Check sheet for the drawn part. Datum: minimum x, y, z corner. Units: mm. A direction names the side the tool comes from. Round coordinates to 2 decimals unless told otherwise and drop trailing zeros. Write each loop counter-clockwise with the first axis right and the second up, starting at its lowest first coordinate (ties: lowest second). Pieces come first, ordered by that corner, then holes. Notation, with made-up numbers: M 71.5,81 L 81.5,81 A23 cw 81.5,108 Z; hole C -22.5,58 d11. An arc over 180 degrees is marked long. Answer in a Markdown table with one row per item. Add a question column.
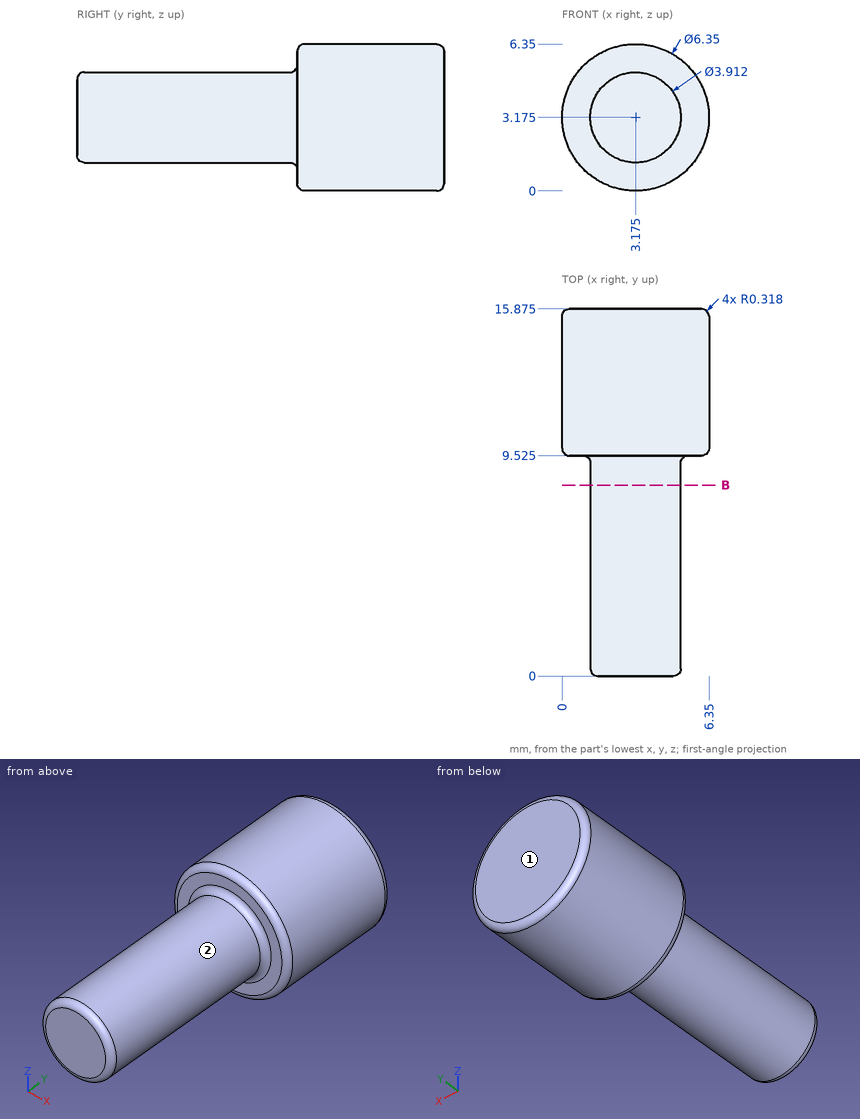
Item 1: Section check B-B, the plane y = 8.25. Record the boundary of the cut face in (x, z) (1 decimal).
Item 2: Scan lines: probe 1 along Y at (x, z) = (1.25, 4.5) (1 decimal); probe 2 along X at (y, z) = (11.5, 3.25); probe 3 along Z at (x, y) = (3.25, 5.25). Record each from-to range of solid material in increasing order. Write a range as from..to.
Item 3: Gauge pin test, flat ends, axial feed: pin 1 Ø3 at (y, z) = (9, 5) entering from -X; pin 2 Ø2 at (y, z) = (8, 1) entering from +X. Record the tip position at first contact, or that the pin passes through.
Item 4: Access from +Z, -Z, +X, -X, +Y, -Y to the whole of each face (thin tool, end or side, straight path). Record for the marked faces 1 and 2.
Result sheet:
| question | item | result |
|---|---|---|
| 1 | outline | C 3.2,3.2 d3.9 |
| 2 | probe 1 | y = 9.5..15.9 |
| 2 | probe 2 | x = 0..6.35 |
| 2 | probe 3 | z = 1.22..5.13 |
| 3 | pin 1 | stops at x = 0.05 |
| 3 | pin 2 | stops at x = 4.74 |
| 4 | face 1 | +Z, -Z, +X, -X, +Y |
| 4 | face 2 | -Y |
